```python
from build123d import *

# Parameters (mm, degrees)
BOSS_EXTRUDE1_DEPTH                               = 10.16
CSK_FOR_8_FLAT_HEAD_MACHINE_SCREW_100_D           = 4.9149
CSK_FOR_8_FLAT_HEAD_MACHINE_SCREW_100_CSINK_D     = 8.4328
CSK_FOR_8_FLAT_HEAD_MACHINE_SCREW_100_CSINK_ANGLE = 100
SKETCH5_W                                         = 16.54
SKETCH5_H                                         = 3.175
CUT_EXTRUDE1_DEPTH                                = 51.038
SKETCH6_W                                         = 12.7
SKETCH6_H                                         = 0.5
BOSS_EXTRUDE2_DEPTH                               = 5.334


with BuildPart() as part:
    # Sketch1 → Boss-Extrude1 (new body)
    with BuildSketch(Plane(origin=(0, 19.05, 0), x_dir=(1, 0, 0), z_dir=(0, 1, 0))):
        Polygon((15.54, 76.2), (15.54, 44.45), (28.24, 44.45), (28.24, 88.9), (-28.24, 88.9), (-28.24, 38.862), (-15.54, 38.862), (-15.54, 76.2), align=None)
    extrude(amount=BOSS_EXTRUDE1_DEPTH)

    # CSK for #8 Flat Head Machine Screw (100)1 (through all)
    with Locations(Plane(origin=(0, 29.21, 0), x_dir=(1, 0, 0), z_dir=(0, 1, 0))):
        with Locations((-21.89, 82.55), (21.89, 82.55), (-21.89, 45.212), (21.89, 50.8)):
            CounterSinkHole(CSK_FOR_8_FLAT_HEAD_MACHINE_SCREW_100_D / 2, CSK_FOR_8_FLAT_HEAD_MACHINE_SCREW_100_CSINK_D / 2, counter_sink_angle=CSK_FOR_8_FLAT_HEAD_MACHINE_SCREW_100_CSINK_ANGLE)

    # Sketch5 → Cut-Extrude1 (cut, through all)
    with BuildSketch(Plane(origin=(0, 0, -88.9), x_dir=(-1, 0, 0), z_dir=(0, 0, -1))):
        with Locations((0.015, 27.6225)):
            Rectangle(SKETCH5_W, SKETCH5_H)
    extrude(amount=-CUT_EXTRUDE1_DEPTH, mode=Mode.SUBTRACT)

    # Sketch6 → Boss-Extrude2 (add)
    with BuildSketch(Plane.XZ.offset(-19.05)):
        with Locations((-21.89, -38.612)):
            Rectangle(SKETCH6_W, SKETCH6_H)
        Polygon((-28.24, -32.012), (-28.24, -38.362), (-15.54, -38.362), (-8.89, -38.362), (-8.89, -32.012), align=None)
        with Locations((21.89, -44.2)):
            Rectangle(SKETCH6_W, SKETCH6_H)
        Polygon((8.89, -43.95), (15.54, -43.95), (28.24, -43.95), (28.24, -37.6), (8.89, -37.6), align=None)
    extrude(amount=-BOSS_EXTRUDE2_DEPTH)


solid = part.part
```
The model under review builds one solid part; all positions refer to its coordinate system, in mm. A direction names the side the tool comes from. Round coordinates to 2 decimals unless told otherwise and drop trailing zeros. Loops run counter-clockwise (first coordinate to the right, second up) from the corner with the lowest first, then second, coordinate; pieces in that order, holes last. Notation, with made-up numbers: (4.5, 5) - (27.5, 5) arc R27 ccw to (27.5, 44) - close; hole circle Ø5 at (18.25, 12). An arc over 180 degrees is marked (long way). Use a Markdown table: item, result. Add a question column.
Q1. The part is to be moulded in two halves that separate along Z. For faces 5 (the face through (-21.57, 23.33, -47.65)), 6 (the face through (-28.24, 24, -60)), 7 (the face through (-18, 22, -32.012)), say which applies: pulls with the +Z half, pulls with the -Z half, needs draft (parallel to the pull), parting line crosses it, or undercut.
Q2. Add section D-D (z = -50.8). State the section outline as (x, y) points.
Q3. Insertion check: pin 1 Ø5.5 at (x, z) = (17.5, -39.5) entering from +Y; pin 2 Ø14 at (x, z) = (-3, -82) entering from +Y; pin 3 Ø5.5 at (x, y) = (19, 28) entering from +Z; pin 4 Ø5.5 at (x, z) = (21.89, -50.8) entering from +Y. Each pin has a flat end and moves straight along its axis. Give the tip position at first contact, or say it passes through.
Q4. Add section B-B (x = 21.89). State the section outline as (y, z) points.
Q5. Add section A-A (z = -82.55). State the section outline as (x, y) points (3 decimals).
Q6. Add section C-C (y = 23.5). State the section outline as (x, z) points.
Q7. Machinability: for faces 1 (the face through (8.255, 28, -83)), 2 (the face through (8.89, 22, -41)), 3 (the face through (18, 24.384, -41)), 4 (the face through (-22, 27, -38.862)), which of the approach directions +Z, -Z, +X, -X, +Y, -Y give a long, thin tool a straight path to every point of the face, cutting with its end or side? Answer none if there is none.
Q8. For probe 1 along X at (y, z) = (23, -82.55); probe 2 along Z at (x, y) = (21.89, 25); probe 3 along X at (y, z) = (28, -64), list the stretches that pass through material, from the lowest coordinate up.
Worked answers:
| question | item | result |
|---|---|---|
| 1 | face 5 | undercut |
| 1 | face 6 | needs draft |
| 1 | face 7 | pulls with the +Z half |
| 2 | outline | (-28.24, 19.05) - (-15.54, 19.05) - (-15.54, 29.21) - (-28.24, 29.21) - close; (15.54, 19.05) - (19.43, 19.05) - (19.43, 27.73) - (17.67, 29.21) - (15.54, 29.21) - close; (24.35, 19.05) - (28.24, 19.05) - (28.24, 29.21) - (26.11, 29.21) - (24.35, 27.73) - close |
| 3 | pin 1 | y = 24.38 |
| 3 | pin 2 | y = 29.21 |
| 3 | pin 3 | z = -44.45 |
| 3 | pin 4 | y = 27.98 |
| 4 | outline | (19.05, -88.9) - (29.21, -88.9) - (29.21, -86.77) - (27.73, -85.01) - (19.05, -85.01) - close; (19.05, -80.09) - (27.73, -80.09) - (29.21, -78.33) - (29.21, -55.02) - (27.73, -53.26) - (19.05, -53.26) - close; (19.05, -48.34) - (27.73, -48.34) - (29.21, -46.58) - (29.21, -44.45) - (24.38, -44.45) - (24.38, -37.6) - (19.05, -37.6) - close |
| 5 | outline | (-28.24, 19.05) - (-24.347, 19.05) - (-24.347, 27.734) - (-26.106, 29.21) - (-28.24, 29.21) - close; (-19.433, 19.05) - (19.433, 19.05) - (19.433, 27.734) - (17.674, 29.21) - (8.255, 29.21) - (8.255, 26.035) - (-8.285, 26.035) - (-8.285, 29.21) - (-17.674, 29.21) - (-19.433, 27.734) - close; (24.347, 19.05) - (28.24, 19.05) - (28.24, 29.21) - (26.106, 29.21) - (24.347, 27.734) - close |
| 6 | outline | (-28.24, -88.9) - (28.24, -88.9) - (28.24, -37.6) - (8.89, -37.6) - (8.89, -43.95) - (15.54, -43.95) - (15.54, -76.2) - (-15.54, -76.2) - (-15.54, -38.36) - (-8.89, -38.36) - (-8.89, -32.01) - (-28.24, -32.01) - close; hole circle Ø4.91 at (-21.89, -82.55); hole circle Ø4.91 at (-21.89, -45.21); hole circle Ø4.91 at (21.89, -82.55); hole circle Ø4.91 at (21.89, -50.8) |
| 7 | face 1 | +Z, -Z, +Y |
| 7 | face 2 | +Z, +Y, -Y |
| 7 | face 3 | +Z, +X, +Y |
| 7 | face 4 | +Z, +X, -X, +Y |
| 8 | probe 1 | -28.24 to -24.35, -19.43 to 19.43, 24.35 to 28.24 |
| 8 | probe 2 | -88.9 to -85.01, -80.09 to -53.26, -48.34 to -44.45 |
| 8 | probe 3 | -28.24 to -15.54, 15.54 to 28.24 |
